The figure shows three views and two pictorial views of one solid part (mm, origin at its lowest corner). Answer the questions. A direction names the side the tool comes from. Round coordinates to 2 decimals unless told otherwise and drop trailing zeros. Order: outer loops, then holes, each group sorted by start corner. A loop starts at its lowest first (then second) coordinate and runs counter-clockwise, first axis right, second up. Notation, with made-up numbers: (61, 16) - (88, 16) arc R35 ccw to (88, 55) - close; hole circle Ø9 at (-24.75, -24.5). An arc over 180 degrees is marked (long way). Answer in a Markdown table with one row per item.
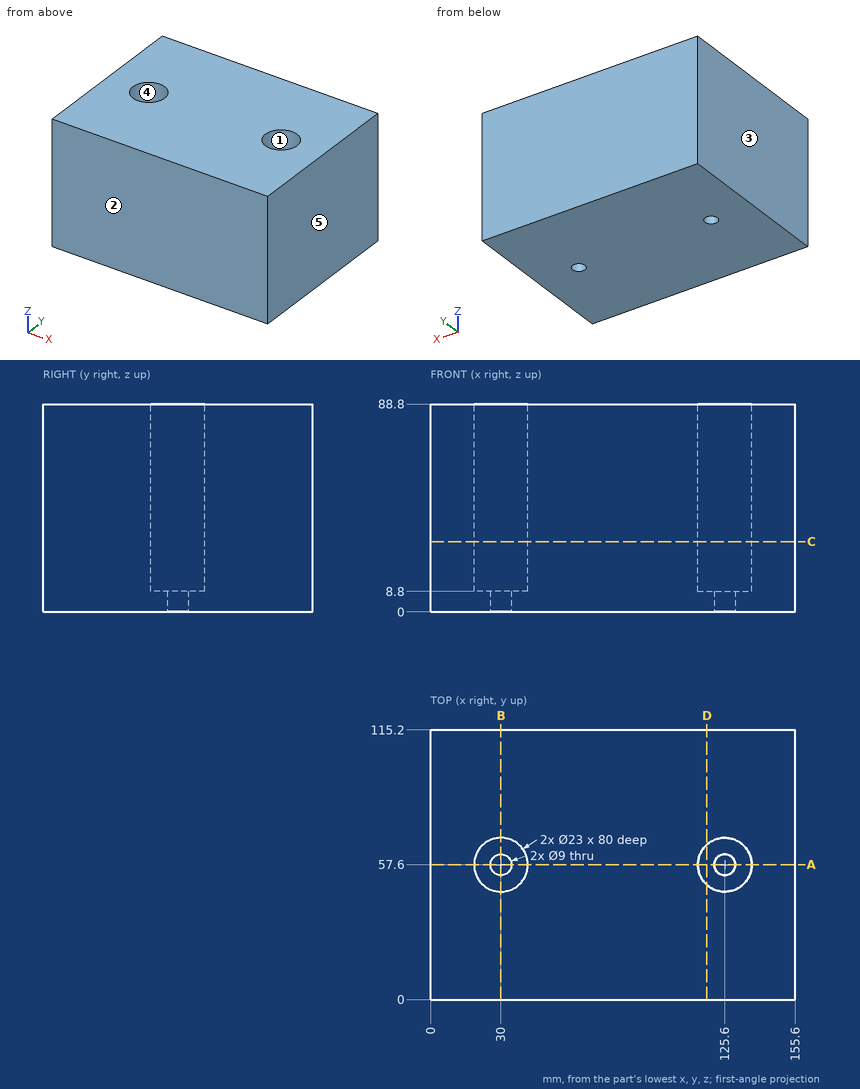
1) Find section C-C, the plane z = 30. Give the vertices of the cut face in (x, y).
Filled in:
| item | result |
|---|---|
| outline | (0, 0) - (155.6, 0) - (155.6, 115.2) - (0, 115.2) - close; hole circle Ø23 at (30, 57.6); hole circle Ø23 at (125.6, 57.6) |
2) Each of these flat-tipped pins is pushed along its axis until it touches: pin 1 (5 mm diameter, centred on x = 121.5, z = 54.5, fed in from -Y); pin 2 (11.5 mm diameter, centred on x = 28.5, y = 62.5, fed in from +Z). Where does it stop, or does it pass through?
Filled in:
| item | result |
|---|---|
| pin 1 | stops at y = 0 |
| pin 2 | stops at z = 8.8 |
3) Which of the six approach directions +Z, -Z, +X, -X, +Y, -Y give full straight-line access (tool end or side, diameter ignored) to the marked faces 4 and 5?
Filled in:
| item | result |
|---|---|
| face 4 | +Z |
| face 5 | +Z, -Z, +X, +Y, -Y |
4) Find section A-A, the plane y = 57.6. Give the vertices of the cut face in (x, z), then the cut area to 3 significant figures.
Filled in:
| item | result |
|---|---|
| outline | (0, 0) - (25.5, 0) - (25.5, 8.8) - (18.5, 8.8) - (18.5, 88.8) - (0, 88.8) - close; (34.5, 0) - (121.1, 0) - (121.1, 8.8) - (114.1, 8.8) - (114.1, 88.8) - (41.5, 88.8) - (41.5, 8.8) - (34.5, 8.8) - close; (130.1, 0) - (155.6, 0) - (155.6, 88.8) - (137.1, 88.8) - (137.1, 8.8) - (130.1, 8.8) - close |
| area | 9,980 mm^2 |
5) Find section B-B, the plane x = 30. Give the vertices of the cut face in (y, z), then the cut area to 3 significant figures.
Filled in:
| item | result |
|---|---|
| outline | (0, 0) - (53.1, 0) - (53.1, 8.8) - (46.1, 8.8) - (46.1, 88.8) - (0, 88.8) - close; (62.1, 0) - (115.2, 0) - (115.2, 88.8) - (69.1, 88.8) - (69.1, 8.8) - (62.1, 8.8) - close |
| area | 8,310 mm^2 |
6) Find the intervals of material crossed by probe 1 along X at (y, z) = (57, 61); probe 2 along Y at (x, z) = (30, 3); probe 3 along X at (y, z) = (63, 69), in increasing order. Write a range as from..to.
Filled in:
| item | result |
|---|---|
| probe 1 | x = 0..18.52, 41.48..114.12, 137.08..155.6 |
| probe 2 | y = 0..53.1, 62.1..115.2 |
| probe 3 | x = 0..19.85, 40.15..115.45, 135.75..155.6 |
7) The mould has two halves that part along X. Classify the marked faces 1, 2 and 3: released by +X, released by -X, zero draft, split by the parting line, or undercut.
Filled in:
| item | result |
|---|---|
| face 1 | undercut |
| face 2 | zero draft |
| face 3 | released by -X |
8) Find section D-D, the plane x = 118. Give the vertices of the cut face in (y, z).
Filled in:
| item | result |
|---|---|
| outline | (0, 0) - (115.2, 0) - (115.2, 88.8) - (66.23, 88.8) - (66.23, 8.8) - (48.97, 8.8) - (48.97, 88.8) - (0, 88.8) - close |
